Part model, mm, in its own coordinate system. Give positions to 0.01 mm unless a question says otherwise; leave off trailing zeros. Order: outer loops, then holes, each group sorted by start corner. A loop starts at its lowest first (then second) coordinate and runs counter-clockwise, first axis right, second up. Notation, with made-up numbers: (32, -15) - (73, -15) arc R20 ccw to (73, 15) - close; hole circle Ø1 at (9.5, 45). An arc over 180 degrees is marked (long way). Use one line per item in the form item = value. Start each with the question number.
1. Pull direction X, two halves, no side cores. Call faces 1 (the face through (0, 30, 0)), 2 (the face through (0.66, 32.958, -14.985)), 3 (the face through (-11.609, 32.958, 4.413)): +X half, -X half, draft (parallel to the pull), parting line (faces both ways), or undercut.
2. Pin check, flat tips, straight feed: P1, Ø1, axis at x = -4, y = 32.5, coming from the +Z side; P2, Ø1, axis at x = -7, y = 33, coming from the -Z side; P3, Ø1.5, axis at x = -9.5, y = 33.5, coming from the -Z side; P4, Ø1, axis at x = -0.5, y = 34.5, coming from the -Z side. Stop position of each tip, or through.
3. Band-saw the part on C-C, the plane y = 32.9. List the corners of the cut face in (x, z).
4. Band-saw the part on B-B, the plane x = 0. List the corners of the cut face in (y, z), plus the area to 3 significant figures.
5. Band-saw the part on A-A, the plane z = 12. List the corners of the cut face in (x, y), plus the area to 3 significant figures.
6. Band-saw the part on D-D, the plane z = 6. List the corners of the cut face in (x, y), plus the area to 3 significant figures.
7. Drill centre lines: line 1 (Z direction, x = 9.5, y = 31.3); line 2 (X direction, y = 33.8, z = -6); line 3 (X direction, y = 31.05, z = 4.25). Where is each one in solid material? Low to high.
from build123d import *

# Parameters (mm, degrees)
SKETCH1_R             = 15
BOSS_EXTRUDE1_DEPTH   = 30
SKETCH2_R             = 7
BOSS_EXTRUDE2_DEPTH   = 4
F_4_0MM_DOWEL_HOLE1_D = 4
CIRPATTERN1_COUNT     = 6
SKETCH6_R             = 15
SKETCH6_R_2           = 2
BOSS_EXTRUDE3_DEPTH   = 6


with BuildPart() as part:
    # Sketch1 → Boss-Extrude1 (new body)
    with BuildSketch(Plane(origin=(0, 0, 0), x_dir=(1, 0, 0), z_dir=(0, 1, 0))):
        with Locations(Location((0, 0, 0), (0, 0, 270))):
            Circle(SKETCH1_R)
    extrude(amount=BOSS_EXTRUDE1_DEPTH)

    # Sketch2 → Boss-Extrude2 (add)
    with BuildSketch(Plane.XZ):
        with Locations(Location((0, 0, 0), (0, 0, 270))):
            Circle(SKETCH2_R)
    extrude(amount=BOSS_EXTRUDE2_DEPTH)

    # Ø4.0mm Dowel Hole1 (through all)
    with Locations(Plane(origin=(0, 0, 0), x_dir=(-1, 0, 0), z_dir=(0, -1, 0))):
        with Locations((0, -12)):
            f_4_0mm_dowel_hole1 = Hole(F_4_0MM_DOWEL_HOLE1_D / 2)

    # CirPattern1: Ø4.0mm Dowel Hole1 ×6 about axis
    cirpattern1_axis = Axis((0, 0, 0), (0, 1, 0))
    for i in range(1, CIRPATTERN1_COUNT):
        add(f_4_0mm_dowel_hole1.rotate(cirpattern1_axis, i * 360 / CIRPATTERN1_COUNT), mode=Mode.SUBTRACT)


with BuildPart() as body_2:
    # Sketch6 → Boss-Extrude3 (new body)
    with BuildSketch(Plane(origin=(0, 30, 0), x_dir=(1, 0, 0), z_dir=(0, 1, 0))):
        with Locations(Location((0, 0, 0), (0, 0, 270))):
            Circle(SKETCH6_R)
        with Locations(Location((-10.392304845, 6, 0), (0, 0, 270))):
            Circle(SKETCH6_R_2, mode=Mode.SUBTRACT)
        with Locations(Location((-10.392304845, -6, 0), (0, 0, 270))):
            Circle(SKETCH6_R_2, mode=Mode.SUBTRACT)
        with Locations(Location((0, -12, 0), (0, 0, 270))):
            Circle(SKETCH6_R_2, mode=Mode.SUBTRACT)
        with Locations(Location((10.392304845, -6, 0), (0, 0, 270))):
            Circle(SKETCH6_R_2, mode=Mode.SUBTRACT)
        with Locations(Location((10.392304845, 6, 0), (0, 0, 270))):
            Circle(SKETCH6_R_2, mode=Mode.SUBTRACT)
        with Locations(Location((0, 12, 0), (0, 0, 270))):
            Circle(SKETCH6_R_2, mode=Mode.SUBTRACT)
    extrude(amount=BOSS_EXTRUDE3_DEPTH)


solid = body_2.part
From the geometry:
q1.face_1 = draft
q1.face_2 = parting line
q1.face_3 = undercut
q2.P1 = 14.59
q2.P2 = -13.52
q2.P3 = -12.18
q2.P4 = -15
q3.outline = circle Ø30 at (0, 0); hole circle Ø4 at (-10.39, -6); hole circle Ø4 at (-10.39, 6); hole circle Ø4 at (0, -12); hole circle Ø4 at (0, 12); hole circle Ø4 at (10.39, -6); hole circle Ø4 at (10.39, 6)
q4.outline = (30, -15) - (36, -15) - (36, -14) - (30, -14) - close; (30, -10) - (36, -10) - (36, 10) - (30, 10) - close; (30, 14) - (36, 14) - (36, 15) - (30, 15) - close
q4.area = 132 mm²
q5.outline = (-9, 30) - (-2, 30) - (-2, 36) - (-9, 36) - close; (2, 30) - (9, 30) - (9, 36) - (2, 36) - close
q5.area = 84.0 mm²
q6.outline = (-13.75, 30) - (-12.39, 30) - (-12.39, 36) - (-13.75, 36) - close; (-8.39, 30) - (8.39, 30) - (8.39, 36) - (-8.39, 36) - close; (12.39, 30) - (13.75, 30) - (13.75, 36) - (12.39, 36) - close
q6.area = 117 mm²
q7.line_1 = -11.61 to -7.79, -4.21 to 4.21, 7.79 to 11.61
q7.line_2 = -13.75 to -12.39, -8.39 to 8.39, 12.39 to 13.75
q7.line_3 = -14.39 to -11.36, -9.42 to 9.42, 11.36 to 14.39
